Part model, mm, in its own coordinate system. A direction names the side the tool comes from. Give positions to 0.01 mm unless a question says otherwise; leave off trailing zeros. Order: outer loops, then holes, each group sorted by start corner. A loop starts at its lowest first (then second) coordinate and runs counter-clockwise, first axis right, second up.
from build123d import *

# Parameters (mm, degrees)
F1_DEPTH = 32.5
F2_W     = 25
F2_H     = 10
F3_DEPTH = 20.001
F4_SIZE  = 15
F5_R     = 5
F6_DEPTH = 20.001


with BuildPart() as f1:
    # F0 (on Right) → F1 (new body, symmetric)
    with BuildSketch(Plane.YZ):
        Polygon((0, 45), (0, 0), (45, 0), (45, 20), (20, 20), (20, 45), align=None)
    extrude(amount=F1_DEPTH, both=True)

    # F2 (on face) → F3 (cut, through all)
    with BuildSketch(Plane.XY.offset(20)):
        with Locations((0, 40)):
            Rectangle(F2_W, F2_H)
    extrude(amount=-F3_DEPTH, mode=Mode.SUBTRACT)

    # F4
    f4_edges = [f1.edges().sort_by_distance(p)[0] for p in [
        (32.5, 10, 45),
        (-32.5, 10, 45),
    ]]
    chamfer(f4_edges, length=F4_SIZE)

    # F5 (on face) → F6 (cut, through all)
    with BuildSketch(Plane(origin=(0, 20, 0), x_dir=(-1, 0, 0), z_dir=(0, 1, 0))):
        with Locations((0, 32)):
            Circle(F5_R)
    extrude(amount=-F6_DEPTH, mode=Mode.SUBTRACT)


solid = f1.part
Item 1: Pull direction Z, two halves, no side cores. Call faces 4 (the face through (0, 0, 23)), 5 (the face through (24.9, 10.1, 37.6)), 6 (the face through (1.08, 10.14, 27.12)): released by +Z, released by -Z, zero draft, split by the parting line, or undercut.
Item 2: Which spindle directions (+Z, -Z, +X, -X, +Y, -Y) get a long thin tool onto all of the face, cutting with end or side? Do faces 1 (the face through (-24.9, 10.1, 37.6)), 2 (the face through (0, 33, 20)), 3 (the face through (0, 35, 10)). Say none if no direction does.
Item 3: Band-saw the part on A-A on x = 0. List the corners of the cut face in (y, z).
Item 4: Drill centre lines: probe 1 along Z at (x, y) = (0, 11); probe 2 along X at (y, z) = (43, 19.5); probe 3 along Z at (x, y) = (-19, 26). Where is each one in solid material? Low to high.
Item 5: Band-saw the part on D-D on x = -24.5. List the corners of the cut face in (y, z), plus the area to 3 significant figures.
Item 6: Band-saw the part on C-C on z = 12.5. List the corners of the cut face in (x, y), plus the area to 4 significant figures.
Item 7: Drop flat-ended pins along their axis: P1, Ø1, axis at x = -10, z = 16, coming from the +Y side; P2, Ø5, axis at x = 0.5, z = 27, coming from the +Y side; P3, Ø7.5, axis at x = -6, y = 34, coming from the +Z side; P4, Ø6, axis at x = 0, z = 32, coming from the -Y side. Give the stop position or say it passes through.
Item 8: Band-saw the part on B-B on y = 15. List the corners of the cut face in (x, z), plus the area to 3 significant figures.
Working result:
1. face 4: zero draft
1. face 5: released by +Z
1. face 6: undercut
2. face 1: +Z, -X, +Y, -Y
2. face 2: +Z, +X, -X, +Y
2. face 3: +Z, -Z, +Y
3. outline: (0, 0) - (35, 0) - (35, 20) - (20, 20) - (20, 27) - (0, 27) - close; (0, 37) - (20, 37) - (20, 45) - (0, 45) - close
4. probe 1: z = 0 to 27, 37 to 45
4. probe 2: x = -32.5 to -12.5, 12.5 to 32.5
4. probe 3: z = 0 to 20
5. outline: (0, 0) - (45, 0) - (45, 20) - (20, 20) - (20, 38) - (0, 38) - close
5. area: 1,260 mm2
6. outline: (-32.5, 0) - (32.5, 0) - (32.5, 45) - (12.5, 45) - (12.5, 35) - (-12.5, 35) - (-12.5, 45) - (-32.5, 45) - close
6. area: 2,675 mm2
7. P1: stops at y = 35
7. P2: stops at y = 20
7. P3: stops at z = 20
7. P4: passes through
8. outline: (-32.5, 0) - (32.5, 0) - (32.5, 30) - (17.5, 45) - (-17.5, 45) - (-32.5, 30) - close; hole circle Ø10 at (0, 32)
8. area: 2,620 mm2
